```python
from build123d import *

# Parameters (mm, degrees)
SKETCH_1_W          = 120
SKETCH_1_H          = 64
EXTRUDE_1_DEPTH     = 3
SKETCH_2_R          = 1.5
CUT_EXTRUDE_1_DEPTH = 3
FILLET_1_R          = 10
SKETCH_3_W          = 20
SKETCH_3_H          = 20
CUT_EXTRUDE_2_DEPTH = 3
SKETCH_4_R          = 26
CUT_EXTRUDE_3_DEPTH = 3
FILLET_2_R          = 5
FILLET_3_R          = 10
FILLET_4_R          = 10
SKETCH_6_R          = 2.1
CUT_EXTRUDE_5_DEPTH = 6
SKETCH_7_R          = 4.5
CUT_EXTRUDE_6_DEPTH = 3


with BuildPart() as part:
    # 草图1 → 凸台-拉伸1 (new body)
    with BuildSketch(Plane(origin=(0, 0, 0), x_dir=(1, 0, 0), z_dir=(0, 1, 0))):
        Rectangle(SKETCH_1_W, SKETCH_1_H)
    extrude(amount=EXTRUDE_1_DEPTH)

    # 草图2 → 切除-拉伸1 (cut)
    with BuildSketch(Plane(origin=(0, 3, 0), x_dir=(1, 0, 0), z_dir=(0, 1, 0))):
        with Locations(Location((-50, 22, 0), (0, 0, 270))):
            Circle(SKETCH_2_R)
        with Locations(Location((50, 22, 0), (0, 0, 90))):
            Circle(SKETCH_2_R)
    extrude(amount=-CUT_EXTRUDE_1_DEPTH, mode=Mode.SUBTRACT)

    # 圆角1
    fillet_1_edges = [part.edges().sort_by_distance(p)[0] for p in [
        (-60, 1.5, -32),
        (60, 1.5, -32),
    ]]
    fillet(fillet_1_edges, radius=FILLET_1_R)

    # 草图3 → 切除-拉伸2 (cut)
    with BuildSketch(Plane.XZ):
        with Locations((0, -22)):
            Rectangle(SKETCH_3_W, SKETCH_3_H)
    extrude(amount=-CUT_EXTRUDE_2_DEPTH, mode=Mode.SUBTRACT)

    # 草图4 → 切除-拉伸3 (cut)
    with BuildSketch(Plane.XZ):
        with Locations((-60, 32)):
            Circle(SKETCH_4_R)
        with Locations((60, 32)):
            Circle(SKETCH_4_R)
    extrude(amount=-CUT_EXTRUDE_3_DEPTH, mode=Mode.SUBTRACT)

    # 圆角2
    fillet_2_edges = [part.edges().sort_by_distance(p)[0] for p in [
        (-10, 1.5, -12),
        (10, 1.5, -12),
    ]]
    fillet(fillet_2_edges, radius=FILLET_2_R)

    # 圆角3
    fillet_3_edges = [part.edges().sort_by_distance(p)[0] for p in [
        (-60, 1.5, 6),
        (60, 1.5, 6),
    ]]
    fillet(fillet_3_edges, radius=FILLET_3_R)

    # 圆角4
    fillet_4_edges = [part.edges().sort_by_distance(p)[0] for p in [
        (-34, 1.5, 32),
        (34, 1.5, 32),
    ]]
    fillet(fillet_4_edges, radius=FILLET_4_R)

    # 草图6 → 切除-拉伸5 (cut)
    with BuildSketch(Plane(origin=(0, 6, 189.146349293), x_dir=(0, 0, 1), z_dir=(0, 1, 0))):
        with Locations((-209.45594255, -26.921391455)):
            Circle(SKETCH_6_R)
        with Locations((-167.762204108, 28.683304163)):
            Circle(SKETCH_6_R)
    extrude(amount=-CUT_EXTRUDE_5_DEPTH, mode=Mode.SUBTRACT)

    # 草图7 → 切除-拉伸6 (cut)
    with BuildSketch(Plane.XZ):
        with Locations(Location((-26.921391455, -20.309593257, 0), (0, 0, 270))):
            Circle(SKETCH_7_R)
        with Locations(Location((28.683304163, 21.384145185, 0), (0, 0, 270))):
            Circle(SKETCH_7_R)
    extrude(amount=-CUT_EXTRUDE_6_DEPTH, mode=Mode.SUBTRACT)


solid = part.part
```
The model under review builds one solid part; all positions refer to its coordinate system, in mm. A direction names the side the tool comes from. Give positions to 0.01 mm unless a question says otherwise; leave off trailing zeros. Write each loop counter-clockwise with the first axis right and the second up, starting at its lowest first coordinate (ties: lowest second). Pieces come first, ordered by that corner, then holes. Notation, with made-up numbers: (54.25, 15.5) - (72.25, 15.5) arc R35 cw to (72.25, 53.5) - close; hole circle Ø4 at (46.5, 49.25). An arc over 180 degrees is marked (long way). Answer in a Markdown table with one row per item. Add a question column.
1. Draft analysis for pull direction X (two halves, no side actions). For faces 1 (the flat face through (10, 1, -25)), 2 (the flat face through (0, 1, 32)), 3 (the cylindrical face through (57.938, 1.479, 3.498)), 4 (the cylindrical face through (-9, 2, -14)), state which applies: +X half, -X half, draft (parallel to the pull), parting line (faces both ways), or undercut.
2. We need section A-A on y = 1.7. Write out the cut boundary in (x, z).
3. We need section B-B on x = 38. Write out the cut boundary in (y, z).
4. Tool access review of faces 5 (the flat face through (-10, 1, -25)), 6 (the cylindrical face through (-31.498, 1.521, 29.938)): name each direction out of +Z, -Z, +X, -X, +Y, -Y from which nothing blocks a thin tool from reaching the whole face with its end or side.
5. Wall thickness on line 1 along X through (y, z) = (1.4, -17.5); line 2 along X through (y, z) = (1.85, -18.5); line 3 along X through (y, z) = (1.35, -22): over which ranges is each line inside the solid? List them lowest first. Write a range as [from, to].
6. Insertion check: P1, Ø1.8, axis at x = -50, z = -22, coming from the -Y side; P2, Ø1.5, axis at y = 1, z = -25.5, coming from the -X side; P3, Ø0.9, axis at y = 1, z = -25.5, coming from the +X side. Each pin has a flat end and moves straight along its axis. Give the tip position at first contact, or say it passes through.
Ans:
| question | item | result |
|---|---|---|
| 1 | face 1 | undercut |
| 1 | face 2 | draft |
| 1 | face 3 | +X half |
| 1 | face 4 | undercut |
| 2 | outline | (-60, -22) arc R10 ccw to (-50, -32) - (-10, -32) - (-10, -17) arc R5 cw to (-5, -12) - (5, -12) arc R5 cw to (10, -17) - (10, -32) - (50, -32) arc R10 ccw to (60, -22) - (60, -2.58) arc R10 ccw to (52.78, 7.02) arc R26 cw to (35.02, 24.78) arc R10 ccw to (25.42, 32) - (-25.42, 32) arc R10 ccw to (-35.02, 24.78) arc R26 cw to (-52.78, 7.02) arc R10 ccw to (-60, -2.58) - close; hole circle Ø3 at (-50, -22); hole circle Ø9 at (-26.92, -20.31); hole circle Ø9 at (28.68, 21.38); hole circle Ø3 at (50, -22) |
| 3 | outline | (0, -32) - (3, -32) - (3, 18.14) - (0, 18.14) - close |
| 4 | face 5 | -Z, +Y, -Y |
| 4 | face 6 | +Z, -X, +Y, -Y |
| 5 | line 1 | x = [-60, -30.44], [-23.41, -10], [10, 60] |
| 5 | line 2 | x = [-60, -31.04], [-22.8, -10], [10, 60] |
| 5 | line 3 | x = [-60, -51.5], [-48.5, -31.09], [-22.75, -10], [10, 48.5], [51.5, 60] |
| 6 | P1 | passes through |
| 6 | P2 | stops at x = -59.61 |
| 6 | P3 | stops at x = 59.52 |
